Part model, mm, in its own coordinate system. A direction names the side the tool comes from. Round coordinates to 2 decimals unless told otherwise and drop trailing zeros. Loops run counter-clockwise (first coordinate to the right, second up) from the corner with the lowest first, then second, coordinate; pieces in that order, holes last.
(1) Cut at D-D on z = -0.5. Count the separate pieces of the cut face and the enclosed holes in it, then the cut area to 3 significant figures.
(2) Cut at C-C on x = -4.5. List the corners of the cut face in (y, z), then the cut area to 3 significant figures.
(3) Tool access for faces 5 (the face through (1, 0, 4)), 6 (the face through (50, 0.1, 4.5)): list every direction of +Z, -Z, +X, -X, +Y, -Y with a clear straight run to the whole face (end or side of a thin tool).
(4) Mould opens along Y. For faces 1 (the face through (1, 5, 0)), 2 (the face through (36.82, 1.08, 4.51)), 3 (the face through (43.58, 4.51, 0.74)), 4 (the face through (1, 0, -4)) say: +Y half, -Y half, draft (parallel to the pull), parting line (faces both ways), or undercut.
(5) Flat gauge pin, fed straight in: pin 1 (4 mm diameter, centred on y = 0, z = 1, fed in from +X). Where does the tip first touch, or does it go through?
(6) Probe probe 1 along X at (y, z) = (4.5, 0); probe 2 along Y at (x, z) = (-21, 1.75). List the from-to ranges inside material, lowest first.
(7) Cut at A-A on y = -3. List the corners of the cut face in (x, z).
(8) Cut at B-B on x = 38. List the corners of the cut face in (y, z), then the cut area to 3 significant figures.
from build123d import *

# Parameters (mm, degrees)
SKETCH_1_W          = 10
SKETCH_1_H          = 10
EXTRUDE_1_DEPTH     = 50
SKETCH_2_W          = 8
SKETCH_2_H          = 8
CUT_EXTRUDE_1_DEPTH = 101.249688279
SKETCH_3_R          = 1.6
CUT_EXTRUDE_2_DEPTH = 52.23475383
SKETCH_4_R          = 1.6
CUT_EXTRUDE_3_DEPTH = 52.23475383


with BuildPart() as part:
    # ｽｹｯﾁ1 → ﾎﾞｽ - 押し出し1 (new, symmetric)
    with BuildSketch(Plane(origin=(0, 0, 0), x_dir=(0, 0, -1), z_dir=(1, 0, 0))):
        Rectangle(SKETCH_1_W, SKETCH_1_H)
    extrude(amount=EXTRUDE_1_DEPTH, both=True)

    # ｽｹｯﾁ2 → ｶｯﾄ - 押し出し1 (cut, through all)
    with BuildSketch(Plane(origin=(50, 0, 0), x_dir=(0, 0, -1), z_dir=(1, 0, 0))):
        Rectangle(SKETCH_2_W, SKETCH_2_H)
    extrude(amount=-CUT_EXTRUDE_1_DEPTH, mode=Mode.SUBTRACT)

    # ｽｹｯﾁ3 → ｶｯﾄ - 押し出し2 (cut, through all)
    with BuildSketch(Plane(origin=(0, 5, 0), x_dir=(1, 0, 0), z_dir=(0, 1, 0))):
        with Locations(Location((-45, 0, 0), (0, 0, 270))):
            Circle(SKETCH_3_R)
        with Locations(Location((-30, 0, 0), (0, 0, 270))):
            Circle(SKETCH_3_R)
        with Locations(Location((30, 0, 0), (0, 0, 270))):
            Circle(SKETCH_3_R)
        with Locations(Location((45, 0, 0), (0, 0, 270))):
            Circle(SKETCH_3_R)
    extrude(amount=-CUT_EXTRUDE_2_DEPTH, mode=Mode.SUBTRACT)

    # ｽｹｯﾁ4 → ｶｯﾄ - 押し出し3 (cut, through all)
    with BuildSketch(Plane.XY.offset(5)):
        with Locations((-38, 0)):
            Circle(SKETCH_4_R)
        with Locations((38, 0)):
            Circle(SKETCH_4_R)
    extrude(amount=-CUT_EXTRUDE_3_DEPTH, mode=Mode.SUBTRACT)


solid = part.part
Final values:
1. separate pieces: 10
1. enclosed holes: 0
1. area: 176 mm2
2. outline: (-5, -5) - (5, -5) - (5, 5) - (-5, 5) - close; hole (-4, -4) - (4, -4) - (4, 4) - (-4, 4) - close
2. area: 36.0 mm2
3. face 5: +X, -X
3. face 6: +Z, -Z, +X, +Y, -Y
4. face 1: +Y half
4. face 2: undercut
4. face 3: draft
4. face 4: undercut
5. pin 1: passes through
6. probe 1: x = -50 to -46.6, -43.4 to -31.6, -28.4 to 28.4, 31.6 to 43.4, 46.6 to 50
6. probe 2: y = -5 to -4, 4 to 5
7. outline: (-50, -5) - (50, -5) - (50, -4) - (-50, -4) - close; (-50, 4) - (50, 4) - (50, 5) - (-50, 5) - close
8. outline: (-5, -5) - (-1.6, -5) - (-1.6, -4) - (-4, -4) - (-4, 4) - (-1.6, 4) - (-1.6, 5) - (-5, 5) - close; (1.6, -5) - (5, -5) - (5, 5) - (1.6, 5) - (1.6, 4) - (4, 4) - (4, -4) - (1.6, -4) - close
8. area: 29.6 mm2
